Geometry: see drawing. Coordinates: mm, zero at the bounding-box minimum. A direction names the side the tool comes from. Coordinates: 2 decimals unless noted, no trailing zeros. Write each loop counter-clockwise with the first axis right and the second up, starting at its lowest first coordinate (ties: lowest second). Pieces come first, ordered by that corner, then holes. Notation, with made-up numbers: M 47.25,10.25 L 96.25,10.25 A19 ccw 96.25,38.25 Z; hole C 14.5,-37.75 d8. An arc over 180 degrees is marked long. Write item = value, one per line. Start each with the question number.
1. Section query A-A (y = 47). Output: boundary loops of the cut face in (x, z), then the cut area to 3 significant figures.
2. Pin query (flat end, axial travel): pin 1 Ø1 at (x, z) = (22, 8) entering from +Y; pin 2 Ø2.5 at (x, y) = (33.7, 27) entering from +Z; pin 3 Ø4.5 at (x, y) = (13, 47) entering from +Z; pin 4 Ø1 at (x, y) = (24, 42) entering from -Z. Return the tip coordinate at first contact, or that it passes through.
3. Section query C-C (x = 20). Output: boundary loops of the cut face in (y, z), then the cut area to 3 significant figures.
4. Section query B-B (x = 27). Output: boundary loops of the cut face in (y, z).
5. Access query for the marked faces 1, 2 and 3. Directions: +Z, -Z, +X, -X, +Y, -Y. A direction counts if a zero-diameter tool reaches every point of the face in a straight line with its end or side. Return the directions, or none.
6. Section query D-D (z = 2). Output: boundary loops of the cut face in (x, y).
7. Line query: line 1 along Y through (x, z) = (13, 10.1); line 2 along Z through (x, y) = (27.5, 7); line 3 along Y through (x, z) = (26, 13.75). Output: solid intervals per line, ascending.
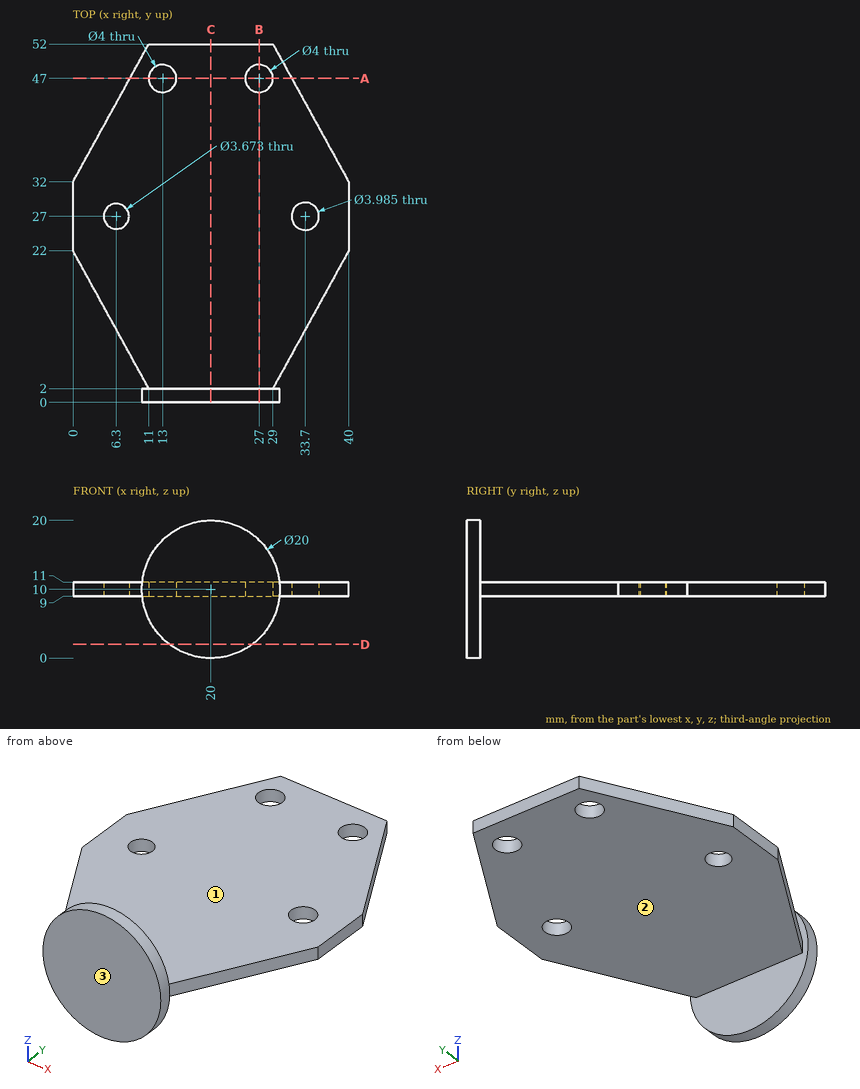
Results are:
q1.outline = M 8.25,9 L 11,9 L 11,11 L 8.25,11 Z; M 15,9 L 25,9 L 25,11 L 15,11 Z; M 29,9 L 31.75,9 L 31.75,11 L 29,11 Z
q1.area = 31.0 mm^2
q2.pin_1 = 2
q2.pin_2 = through
q2.pin_3 = 11
q2.pin_4 = 9
q3.outline = M 0,0 L 2,0 L 2,9 L 52,9 L 52,11 L 2,11 L 2,20 L 0,20 Z
q3.area = 140 mm^2
q4.outline = M 0,2.86 L 2,2.86 L 2,9 L 45,9 L 45,11 L 2,11 L 2,17.14 L 0,17.14 Z; M 49,9 L 52,9 L 52,11 L 49,11 Z
q5.face_1 = +Z, +X, -X, +Y
q5.face_2 = -Z, +X, -X, +Y
q5.face_3 = +Z, -Z, +X, -X, -Y
q6.outline = M 14,0 L 26,0 L 26,2 L 14,2 Z
q7.line_1 = 0 to 45, 49 to 52
q7.line_2 = 9 to 11
q7.line_3 = 0 to 2
